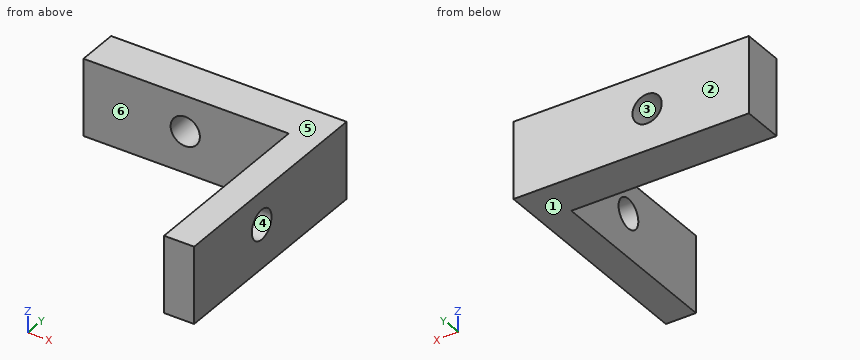
```python
from build123d import *

# Parameters (mm, degrees)
F1_DEPTH = 25.4
F2_R     = 4.889775
F3_DEPTH = 25.4
F4_R     = 4.841352
F5_DEPTH = 14.478


with BuildPart() as f1:
    # F0 (on Top) → F1 (new body)
    with BuildSketch(Plane.XY):
        Polygon((29.374033, 35.010495), (-48.49131, 35.010495), (-48.49131, 21.278509), (19.415045, 21.278509), (19.415045, -40.607721), (29.374033, -40.607721), align=None)
    extrude(amount=F1_DEPTH)

    # F2 (on face) → F3 (cut)
    with BuildSketch(Plane.YZ.offset(29.374033)):
        with Locations((-7.096407, 14.460783)):
            Circle(F2_R)
    extrude(amount=-F3_DEPTH, mode=Mode.SUBTRACT)

    # F4 (on face) → F5 (cut)
    with BuildSketch(Plane(origin=(0, 35.010495, 0), x_dir=(-1, 0, 0), z_dir=(0, 1, 0))):
        with Locations((14.813676, 13.677494)):
            Circle(F4_R)
    extrude(amount=-F5_DEPTH, mode=Mode.SUBTRACT)


solid = f1.part
```
Here's how the part is built. I have some questions about the finished solid (model axes, mm). Face numbers are marked on the shaded views. A direction names the side the tool comes from. Give positions to 0.01 mm unless a question says otherwise; leave off trailing zeros. Order: outer loops, then holes, each group sorted by start corner. A loop starts at its lowest first (then second) coordinate and runs counter-clockwise, first axis right, second up. Notation, with made-up numbers: (33.5, -17.75) - (64.5, -17.75) arc R6 cw to (64.5, -11.75) - close; hole circle Ø1 at (9.5, 17.25). An arc over 180 degrees is marked (long way). Answer as a JSON object with one key per item and string values. Group by question number.
Item 1: If we section it at A-A on z = 11.5: Please give me the cut outline in (x, y).
Item 2: Please list where these lines run through material, in increasing order: probe 1 along Y at (x, z) = (9.5, 8); probe 2 along Z at (x, y) = (-18, 28.5); probe 3 along X at (y, z) = (18, 14.25).
Item 3: If we section it at C-C on x = -16: Please give me the cut outline in (y, z), and give its area (3 significant figures).
Item 4: If we section it at B-B on z = 24.25: Please give me the cut outline in (x, y).
Item 5: If we section it at D-D on y = -15: Please give me the cut outline in (x, z).
Item 6: If we mould it in two halves opening along Z, with no side actions, what happens to the marked faces 1, 2, 3 and 4? For each: pulls with the +Z half, pulls with the -Z half, needs draft (parallel to the pull), parting line crosses it, or undercut.
Item 7: Which directions (+Z, -Z, +X, -X, +Y, -Y) give clear straight access to the entire face, cutting with the end or side of a thin tool? Please do the marked faces 5 and 6.
Item 8: For P1, Ø1, axis at x = 4, z = 16, coming from the -Y side, with a flat end and sliding along its axis, tell me the tip position at first contact or that it passes through.
Result set:
{
 "1": {"outline": "(-48.49, 21.28) - (-19.14, 21.28) - (-19.14, 35.01) - (-48.49, 35.01) - close; (-10.49, 21.28) - (19.42, 21.28) - (19.42, -3.2) - (29.37, -3.2) - (29.37, 35.01) - (-10.49, 35.01) - close; (19.42, -40.61) - (29.37, -40.61) - (29.37, -10.99) - (19.42, -10.99) - close"},
 "2": {"probe 1": "21.28 to 35.01", "probe 2": "0 to 10.03, 17.32 to 25.4", "probe 3": "19.42 to 29.37"},
 "3": {"outline": "(21.28, 0) - (35.01, 0) - (35.01, 8.98) - (21.28, 8.98) - close; (21.28, 18.37) - (35.01, 18.37) - (35.01, 25.4) - (21.28, 25.4) - close", "area": "220 mm²"},
 "4": {"outline": "(-48.49, 21.28) - (19.42, 21.28) - (19.42, -40.61) - (29.37, -40.61) - (29.37, 35.01) - (-48.49, 35.01) - close"},
 "5": {"outline": "(19.42, 0) - (29.37, 0) - (29.37, 25.4) - (19.42, 25.4) - close"},
 "6": {"face 1": "pulls with the -Z half", "face 2": "needs draft", "face 3": "undercut", "face 4": "undercut"},
 "7": {"face 5": "+Z, +X, -X, +Y, -Y", "face 6": "+Z, -Z, -X, -Y"},
 "8": {"P1": "y = 21.28"}
}
